```python
from build123d import *

# Parameters (mm, degrees)
BOSS_EXTRUDE1_DEPTH      = 1200
MIRROR1_START            = -60
MIRROR1_OUTLINE_W        = 2.2
MIRROR1_OUTLINE_H        = 2400
MIRROR1_DEPTH            = 120
MIRROR1_2_OUTLINE_W      = 29.8
MIRROR1_2_OUTLINE_H      = 2400
MIRROR1_2_DEPTH          = 6.3
MIRROR1_START_2          = 53.7
MIRROR1_3_OUTLINE_W      = 29.8
MIRROR1_3_OUTLINE_H      = 2400
MIRROR1_3_DEPTH          = 6.3
FILLET1_R                = 7
M6_CLEARANCE_HOLE1_D     = 7
M6_CLEARANCE_HOLE1_DEPTH = 6.3
LPATTERN1_COUNT          = 3
LPATTERN1_PITCH          = 32.5
LPATTERN1_COUNT_DIR2     = 2
LPATTERN1_PITCH_DIR2     = 52


# Read off the part's stored shape, not the designer's step: Mirror1
with BuildPart() as part:
    # Sketch1 → Boss-Extrude1 (new, symmetric)
    with BuildSketch(Plane.XY):
        Polygon((0, 60), (0, -60), (-32, -60), (-32, -53.7), (-2.2, -53.7), (-2.2, 53.7), (-32, 53.7), (-32, 60), align=None)
    extrude(amount=BOSS_EXTRUDE1_DEPTH, both=True)

    # Mirror1 outline → Mirror1 (add)
    with BuildSketch(Plane(origin=(0, 0, 0), x_dir=(1, 0, 0), z_dir=(0, 1, 0)).offset(MIRROR1_START)):
        with Locations((1.1, 0)):
            Rectangle(MIRROR1_OUTLINE_W, MIRROR1_OUTLINE_H)
    extrude(amount=MIRROR1_DEPTH)

    # Mirror1 2 outline → Mirror1 2 (add)
    with BuildSketch(Plane(origin=(0, 0, 0), x_dir=(1, 0, 0), z_dir=(0, 1, 0)).offset(MIRROR1_START)):
        with Locations((17.1, 0)):
            Rectangle(MIRROR1_2_OUTLINE_W, MIRROR1_2_OUTLINE_H)
    extrude(amount=MIRROR1_2_DEPTH)

    # Mirror1 3 outline → Mirror1 3 (add)
    with BuildSketch(Plane(origin=(0, 0, 0), x_dir=(1, 0, 0), z_dir=(0, 1, 0)).offset(MIRROR1_START_2)):
        with Locations((17.1, 0)):
            Rectangle(MIRROR1_3_OUTLINE_W, MIRROR1_3_OUTLINE_H)
    extrude(amount=MIRROR1_3_DEPTH)

    # Fillet1
    fillet1_edges = [part.edges().sort_by_distance(p)[0] for p in [
        (-2.2, -53.7, 0),
        (-2.2, 53.7, 0),
        (2.2, -53.7, 0),
        (2.2, 53.7, 0),
    ]]
    fillet(fillet1_edges, radius=FILLET1_R)

    # M6 Clearance Hole1
    with Locations(Plane(origin=(0, -60, 0), x_dir=(-1, 0, 0), z_dir=(0, -1, 0))):
        with Locations((-26, -1132.5)):
            m6_clearance_hole1 = Hole(M6_CLEARANCE_HOLE1_D / 2, depth=M6_CLEARANCE_HOLE1_DEPTH)

    # LPattern1: M6 Clearance Hole1 3 × 2
    with Locations(*[(-j * LPATTERN1_PITCH_DIR2, 0, -i * LPATTERN1_PITCH) for i in range(LPATTERN1_COUNT) for j in range(LPATTERN1_COUNT_DIR2) if (i, j) != (0, 0)]):
        add(m6_clearance_hole1, mode=Mode.SUBTRACT)


solid = part.part
```
Model file for the job. Use its own axes, mm. A direction names the side the tool comes from. Coordinates: 2 decimals unless noted, no trailing zeros. Order: outer loops, then holes, each group sorted by start corner. A loop starts at its lowest first (then second) coordinate and runs counter-clockwise, first axis right, second up. Notation, with made-up numbers: (46.5, -33.75) - (72.5, -33.75) arc R18 cw to (72.5, -18.75) - close; hole circle Ø3 at (-32, -9.5). An arc over 180 degrees is marked (long way). Return JSON: item names as keys, results as strings. Group by question number.
1) Tool access for faces 4 (the flat face through (0, 60, -17)), 5 (the flat face through (2.2, -1, 17)): list every direction of +Z, -Z, +X, -X, +Y, -Y with a clear straight run to the whole face (end or side of a thin tool).
2) Mould opens along Y. For faces 1 (the flat face through (-2.2, -1, 17)), 2 (the flat face through (0, -60, -17)), 3 (the flat face through (0, -5, -1200)) say: released by +Y, released by -Y, zero draft, split by the parting line, or undercut.
3) Flat gauge pins, fed straight in: P1, Ø4, axis at x = 26, z = 1067.5, coming from the -Y side; P2, Ø1.5, axis at y = 4, z = -268, coming from the +X side; P3, Ø8, axis at y = -40.5, z = -185.5, coming from the -X side. Where does each tip first touch, or does it go through?
4) Saw through at A-A, the plane z = 117.5. Write the cut outline in (x, y), plus the area to 3 significant figures.
5) Saw through at B-B, the plane y = -19.5. Write the cut outline in (x, z), plus the area to 3 significant figures.
6) Probe line 1 (Z direction, x = 26, y = -56); line 2 (Y direction, x = -10, z = -679); line 3 (Y direction, x = -7.5, z = 1046). List the from-to ranges inside material, lowest first. Write a range as from..to.
Values found:
{
 "1": {"face 4": "+Z, -Z, +X, -X, +Y", "face 5": "+Z, -Z, +X"},
 "2": {"face 1": "undercut", "face 2": "released by -Y", "face 3": "zero draft"},
 "3": {"P1": "stops at y = 53.7", "P2": "stops at x = 2.2", "P3": "stops at x = -2.2"},
 "4": {"outline": "(-32, -60) - (32, -60) - (32, -53.7) - (9.2, -53.7) arc R7 cw to (2.2, -46.7) - (2.2, 46.7) arc R7 cw to (9.2, 53.7) - (32, 53.7) - (32, 60) - (-32, 60) - (-32, 53.7) - (-9.2, 53.7) arc R7 cw to (-2.2, 46.7) - (-2.2, -46.7) arc R7 cw to (-9.2, -53.7) - (-32, -53.7) - close", "area": "1,320 mm²"},
 "5": {"outline": "(-2.2, -1200) - (2.2, -1200) - (2.2, 1200) - (-2.2, 1200) - close", "area": "10,600 mm²"},
 "6": {"line 1": "z = -1200..1064, 1071..1096.5, 1103.5..1129, 1136..1200", "line 2": "y = -60..-53.7, 53.7..60", "line 3": "y = -60..-53.49, 53.49..60"}
}
